Input: dimensioned drawing with shaded views. Units: mm. Origin: part minimum x, y, z. Round coordinates to 2 decimals unless told otherwise and drop trailing zeros. Write each loop counter-clockwise with the first axis right and the second up, starting at its lowest first coordinate (ties: lowest second). Pieces come first, ordered by that corner, then holes. Notation, with made-up numbers: M 84,27.5 L 112,27.5 A37 cw 112,63.5 Z; hole C 76,79 d5. An arc over 180 degrees is marked long. Answer in a Markdown table with one row per item. Add a question column.
Item 1: Cut plane C-C on y = 73.5. Return loops of the section in (x, z).
Item 2: Material intervals for probe 1 along X at (y, z) = (21.5, 5.25); probe 2 along Y at (x, z) = (68.5, 3.5); probe 3 along X at (y, z) = (76.5, 2), sorted ascending.
Item 3: Cut plane B-B on x = 10. Return loops of the section in (y, z), and give its area (3 significant figures).
Item 4: Cut plane D-D on x = 81.5. Return loops of the section in (y, z).
Item 5: Contact query for flat-ended pins moving along their axis: pin 1 (2 mm diameter, centred on y = 25.5, z = 3.5, fed in from +X); pin 2 (2.5 mm diameter, centred on y = 32, z = 4, fed in from -X); pin 3 (2 mm diameter, centred on x = 24.5, z = 5.5, fed in from +Y); pin 4 (4 mm diameter, centred on x = 74.5, z = 4.5, fed in from +Y). Output: stop coordinate, or through.
Item 6: Cut plane A-A on y = 48. Return loops of the section in (x, z), and give its area (3 significant figures).
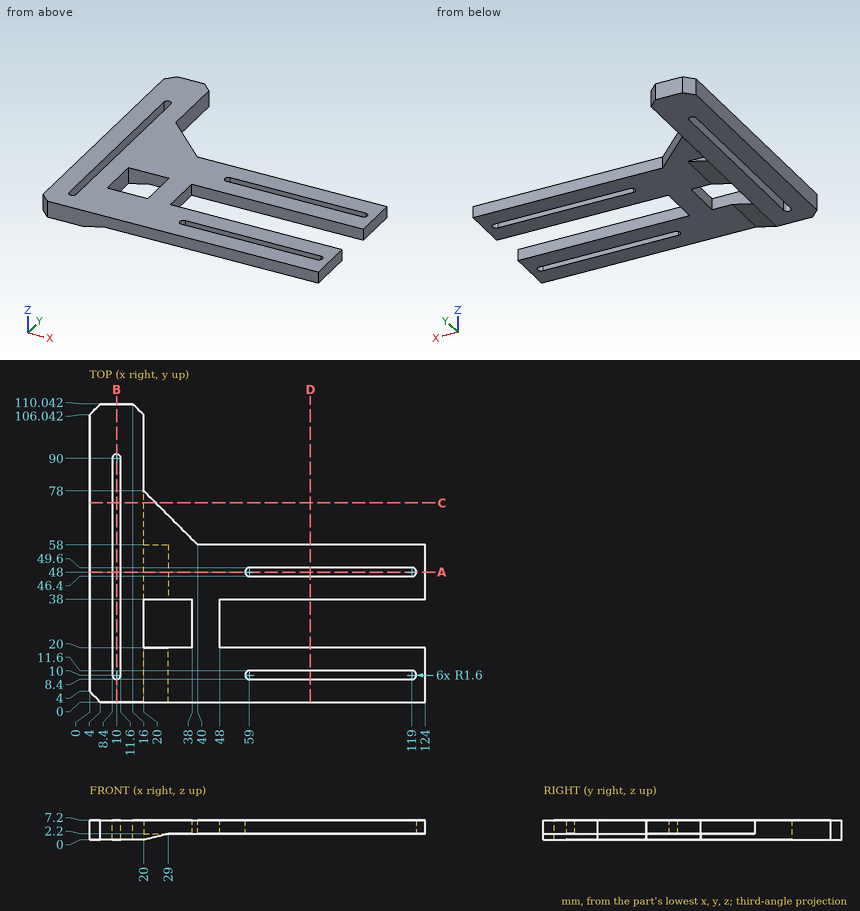
Results below:
| question | item | result |
|---|---|---|
| 1 | outline | M 0,0 L 8.4,0 L 8.4,7.2 L 0,7.2 Z; M 11.6,0 L 20,0 L 20,2.2 L 24.5,2.2 L 24.5,7.2 L 11.6,7.2 Z |
| 2 | probe 1 | 0 to 8.4, 11.6 to 20, 38 to 48 |
| 2 | probe 2 | 0 to 8.4, 11.6 to 20, 38 to 46.4, 49.6 to 58 |
| 2 | probe 3 | 0 to 8.4, 11.6 to 20 |
| 3 | outline | M 0,0 L 8.4,0 L 8.4,7.2 L 0,7.2 Z; M 91.6,0 L 110.04,0 L 110.04,7.2 L 91.6,7.2 Z |
| 3 | area | 193 mm2 |
| 4 | outline | M 0,2.2 L 8.4,2.2 L 8.4,7.2 L 0,7.2 Z; M 11.6,2.2 L 20,2.2 L 20,7.2 L 11.6,7.2 Z; M 38,2.2 L 46.4,2.2 L 46.4,7.2 L 38,7.2 Z; M 49.6,2.2 L 58,2.2 L 58,7.2 L 49.6,7.2 Z |
| 5 | pin 1 | x = 48 |
| 5 | pin 2 | x = 0 |
| 5 | pin 3 | y = 74.5 |
| 5 | pin 4 | y = 58 |
| 6 | outline | M 0,0 L 8.4,0 L 8.4,7.2 L 0,7.2 Z; M 11.6,0 L 20,0 L 29,2.2 L 57.4,2.2 L 57.4,7.2 L 11.6,7.2 Z; M 120.6,2.2 L 124,2.2 L 124,7.2 L 120.6,7.2 Z |
| 6 | area | 335 mm2 |
